Can you work these out from the model? Positions are in its coordinate system, mm. Coordinates: 2 decimals unless noted, no trailing zeros. Write each loop counter-clockwise with the first axis right and the second up, starting at its lowest first coordinate (ties: lowest second). Pieces come first, ordered by that corner, then holes. Notation, with made-up numbers: (37.25, 38) - (57.25, 38) arc R15 cw to (57.25, 47) - close; hole circle Ø4 at (42, -7.5). An arc over 180 degrees is marked (long way). Use one line per item in the form item = value. Start each with the question number.
(1) For pin 1 Ø2 at (x, z) = (-302, -1) entering from +Y; pin 2 Ø14 at (y, z) = (840.5, 18) entering from +X; pin 3 Ø12 at (x, y) = (189.5, 486) entering from +Z; pin 4 Ø2 at (y, z) = (-546.5, 37) entering from +X, each with a flat end and sliding along its axis, tell me the tip position at first contact or that it passes through.
(2) If we section it at A-A on y = -338.5: Please give me the cut outline in (x, z).
(3) If we section it at B-B on z = 18: Give the number of separate pieces and of enclosed holes in the cut face, then the cut area to 3 significant figures.
(4) Thinking about a two-plate mould opening in Y: for faces 1 (the face through (-4, 17, 0)), 2 (the face through (-4, 17, -2)), which applies, pulls with the +Y half, pulls with the -Y half, needs draft (parallel to the pull), parting line crosses it, or undercut?
(5) If we section it at C-C on x = 154: Please give me the cut outline in (y, z), then the cut area to 3 significant figures.
(6) If I drill on probe 1 along X at (y, z) = (146, 30); probe 2 along Y at (x, z) = (214.5, 6); probe 3 along X at (y, z) = (1013, 0.5), over which ranges is the centre line in solid material (lowest first)? Write a range as from..to.
```python
from build123d import *

# Parameters (mm, degrees)
SKETCH1_W                      = 608
SKETCH1_H                      = 2432
BASE_FLANGE1_DEPTH             = 2
EDGE_FLANGE5_STRIP_W           = 13
EDGE_FLANGE5_STRIP_H           = 2
EDGE_FLANGE5_STRIP_CUT_DEPTH   = 608
EDGE_FLANGE5_STRIP_2_W         = 13
EDGE_FLANGE5_STRIP_2_H         = 2
EDGE_FLANGE5_STRIP_CUT_2_DEPTH = 608
EDGE_FLANGE5_DEPTH             = 608
EDGE_FLANGE5_BEND_DEPTH        = 608
EDGE_FLANGE1_STRIP_W           = 13
EDGE_FLANGE1_STRIP_H           = 2
EDGE_FLANGE1_STRIP_CUT_DEPTH   = 2423
EDGE_FLANGE1_STRIP_2_W         = 13
EDGE_FLANGE1_STRIP_2_H         = 2
EDGE_FLANGE1_STRIP_CUT_2_DEPTH = 2423
EDGE_FLANGE1_DEPTH             = 2423
EDGE_FLANGE1_BEND_DEPTH        = 2423
EDGE_FLANGE3_STRIP_W           = 9.4732
EDGE_FLANGE3_STRIP_H           = 2
EDGE_FLANGE3_STRIP_CUT_DEPTH   = 2423
EDGE_FLANGE3_STRIP_2_W         = 9.4732
EDGE_FLANGE3_STRIP_2_H         = 2
EDGE_FLANGE3_STRIP_CUT_2_DEPTH = 2423
EDGE_FLANGE3_DEPTH             = 2423
EDGE_FLANGE3_BEND_DEPTH        = 2423
SKETCH35_R                     = 6
CUT_EXTRUDE1_DEPTH             = 1361.060292781
LPATTERN1_COUNT                = 16
LPATTERN1_PITCH                = 152
SKETCH37_R                     = 6
CUT_EXTRUDE3_DEPTH             = 2754.099344375
LPATTERN3_COUNT                = 4
LPATTERN3_PITCH                = 152


# Sheet-metal steps are written as plain solids
with BuildPart() as part:
    # Sketch1 → Base-Flange1 (new body)
    with BuildSketch(Plane.XY):
        Rectangle(SKETCH1_W, SKETCH1_H)
    extrude(amount=-BASE_FLANGE1_DEPTH)

    # Edge-Flange5 strip (across the edge) → Edge-Flange5 strip cut (cut)
    with BuildSketch(Plane(origin=(304, 1216, 0), x_dir=(0, -1, 0), z_dir=(-1, 0, 0))):
        with Locations((-2, -1)):
            Rectangle(EDGE_FLANGE5_STRIP_W, EDGE_FLANGE5_STRIP_H)
    extrude(amount=EDGE_FLANGE5_STRIP_CUT_DEPTH, mode=Mode.SUBTRACT)

    # Edge-Flange5 strip 2 (across the edge) → Edge-Flange5 strip cut 2 (cut)
    with BuildSketch(Plane(origin=(-304, -1216, 0), x_dir=(0, 1, 0), z_dir=(1, 0, 0))):
        with Locations((-2, -1)):
            Rectangle(EDGE_FLANGE5_STRIP_2_W, EDGE_FLANGE5_STRIP_2_H)
    extrude(amount=EDGE_FLANGE5_STRIP_CUT_2_DEPTH, mode=Mode.SUBTRACT)

    # Edge-Flange5 section (across the edge) → Edge-Flange5 (add)
    with BuildSketch(Plane(origin=(304, 1216, 0), x_dir=(0, -1, 0), z_dir=(-1, 0, 0))):
        with BuildLine():
            Line((0, 2.5), (0, 38))
            Line((0, 38), (2, 38))
            Line((2, 38), (2, 2.5))
            ThreePointArc((2, 2.5), (2.732233047, 0.732233047), (4.5, 0))
            Line((4.5, 0), (4.5, -2))
            ThreePointArc((4.5, -2), (1.318019485, -0.681980515), (0, 2.5))
        make_face()
    extrude(amount=EDGE_FLANGE5_DEPTH)

    # Edge-Flange5 section 2 (across the edge) → Edge-Flange5 bend (add)
    with BuildSketch(Plane(origin=(-304, -1216, 0), x_dir=(0, 1, 0), z_dir=(1, 0, 0))):
        with BuildLine():
            Line((0, 2.5), (0, 38))
            Line((0, 38), (2, 38))
            Line((2, 38), (2, 2.5))
            ThreePointArc((2, 2.5), (2.732233047, 0.732233047), (4.5, 0))
            Line((4.5, 0), (4.5, -2))
            ThreePointArc((4.5, -2), (1.318019485, -0.681980515), (0, 2.5))
        make_face()
    extrude(amount=EDGE_FLANGE5_BEND_DEPTH)

    # Edge-Flange1 strip (across the edge) → Edge-Flange1 strip cut (cut)
    with BuildSketch(Plane(origin=(304, -1211.5, 0), x_dir=(-1, 0, 0), z_dir=(0, 1, 0))):
        with Locations((-2, -1)):
            Rectangle(EDGE_FLANGE1_STRIP_W, EDGE_FLANGE1_STRIP_H)
    extrude(amount=EDGE_FLANGE1_STRIP_CUT_DEPTH, mode=Mode.SUBTRACT)

    # Edge-Flange1 strip 2 (across the edge) → Edge-Flange1 strip cut 2 (cut)
    with BuildSketch(Plane(origin=(-304, 1211.5, 0), x_dir=(1, 0, 0), z_dir=(0, -1, 0))):
        with Locations((-2, -1)):
            Rectangle(EDGE_FLANGE1_STRIP_2_W, EDGE_FLANGE1_STRIP_2_H)
    extrude(amount=EDGE_FLANGE1_STRIP_CUT_2_DEPTH, mode=Mode.SUBTRACT)

    # Edge-Flange1 section (across the edge) → Edge-Flange1 (add)
    with BuildSketch(Plane(origin=(304, -1211.5, 0), x_dir=(-1, 0, 0), z_dir=(0, 1, 0))):
        with BuildLine():
            Line((0, 2.5), (0, 38))
            Line((0, 38), (2, 38))
            Line((2, 38), (2, 2.5))
            ThreePointArc((2, 2.5), (2.732233047, 0.732233047), (4.5, 0))
            Line((4.5, 0), (4.5, -2))
            ThreePointArc((4.5, -2), (1.318019485, -0.681980515), (0, 2.5))
        make_face()
    extrude(amount=EDGE_FLANGE1_DEPTH)

    # Edge-Flange1 section 2 (across the edge) → Edge-Flange1 bend (add)
    with BuildSketch(Plane(origin=(-304, 1211.5, 0), x_dir=(1, 0, 0), z_dir=(0, -1, 0))):
        with BuildLine():
            Line((0, 2.5), (0, 38))
            Line((0, 38), (2, 38))
            Line((2, 38), (2, 2.5))
            ThreePointArc((2, 2.5), (2.732233047, 0.732233047), (4.5, 0))
            Line((4.5, 0), (4.5, -2))
            ThreePointArc((4.5, -2), (1.318019485, -0.681980515), (0, 2.5))
        make_face()
    extrude(amount=EDGE_FLANGE1_BEND_DEPTH)

    # Edge-Flange3 strip (across the edge) → Edge-Flange3 strip cut (cut)
    with BuildSketch(Plane(origin=(302, -1211.5, 38), x_dir=(0, 0, -1), z_dir=(0, 1, 0))):
        with Locations((-2, -1)):
            Rectangle(EDGE_FLANGE3_STRIP_W, EDGE_FLANGE3_STRIP_H)
    extrude(amount=EDGE_FLANGE3_STRIP_CUT_DEPTH, mode=Mode.SUBTRACT)

    # Edge-Flange3 strip 2 (across the edge) → Edge-Flange3 strip cut 2 (cut)
    with BuildSketch(Plane(origin=(-302, 1211.5, 38), x_dir=(0, 0, -1), z_dir=(0, -1, 0))):
        with Locations((-2, -1)):
            Rectangle(EDGE_FLANGE3_STRIP_2_W, EDGE_FLANGE3_STRIP_2_H)
    extrude(amount=EDGE_FLANGE3_STRIP_CUT_2_DEPTH, mode=Mode.SUBTRACT)

    # Edge-Flange3 section (across the edge) → Edge-Flange3 (add)
    with BuildSketch(Plane(origin=(302, -1211.5, 38), x_dir=(0, 0, -1), z_dir=(0, 1, 0))):
        with BuildLine():
            Line((0, 0.7366), (0, 13))
            Line((0, 13), (2, 13))
            Line((2, 13), (2, 0.7366))
            ThreePointArc((2, 0.7366), (2.215745145, 0.215745145), (2.7366, 0))
            Line((2.7366, 0), (2.7366, -2))
            ThreePointArc((2.7366, -2), (0.801531583, -1.198468417), (0, 0.7366))
        make_face()
    extrude(amount=EDGE_FLANGE3_DEPTH)

    # Edge-Flange3 section 2 (across the edge) → Edge-Flange3 bend (add)
    with BuildSketch(Plane(origin=(-302, 1211.5, 38), x_dir=(0, 0, -1), z_dir=(0, -1, 0))):
        with BuildLine():
            Line((0, 0.7366), (0, 13))
            Line((0, 13), (2, 13))
            Line((2, 13), (2, 0.7366))
            ThreePointArc((2, 0.7366), (2.215745145, 0.215745145), (2.7366, 0))
            Line((2.7366, 0), (2.7366, -2))
            ThreePointArc((2.7366, -2), (0.801531583, -1.198468417), (0, 0.7366))
        make_face()
    extrude(amount=EDGE_FLANGE3_BEND_DEPTH)

    # Sketch35 → Cut-Extrude1 (cut, through all)
    with BuildSketch(Plane(origin=(304, 0, 0), x_dir=(0, 0, -1), z_dir=(1, 0, 0))):
        with Locations((-18, -1135.5)):
            Circle(SKETCH35_R)
    cut_extrude1 = extrude(amount=-CUT_EXTRUDE1_DEPTH, mode=Mode.SUBTRACT)

    # LPattern1: Cut-Extrude1 ×16
    with Locations(*[(0, i * LPATTERN1_PITCH, 0) for i in range(1, LPATTERN1_COUNT)]):
        add(cut_extrude1, mode=Mode.SUBTRACT)

    # Sketch37 → Cut-Extrude3 (cut, through all)
    with BuildSketch(Plane(origin=(0, 1216, -1216), x_dir=(1, 0, 0), z_dir=(0, -1, 0))):
        with Locations(Location((228, 1234, 0), (0, 0, 90))):
            Circle(SKETCH37_R)
    cut_extrude3 = extrude(amount=CUT_EXTRUDE3_DEPTH, mode=Mode.SUBTRACT)

    # LPattern3: Cut-Extrude3 ×4
    with Locations(*[(-i * LPATTERN3_PITCH, 0, 0) for i in range(1, LPATTERN3_COUNT)]):
        add(cut_extrude3, mode=Mode.SUBTRACT)


solid = part.part
```
Reported:
q1.pin_1 = 1215.24
q1.pin_2 = 304
q1.pin_3 = 0
q1.pin_4 = 303.9
q2.outline = (-304, 2.5) arc R4.5 ccw to (-299.5, -2) - (299.5, -2) arc R4.5 ccw to (304, 2.5) - (304, 35.26) arc R2.74 ccw to (301.26, 38) - (289, 38) - (289, 36) - (301.26, 36) arc R0.74 cw to (302, 35.26) - (302, 2.5) arc R2.5 cw to (299.5, 0) - (-299.5, 0) arc R2.5 cw to (-302, 2.5) - (-302, 35.26) arc R0.74 cw to (-301.26, 36) - (-289, 36) - (-289, 38) - (-301.26, 38) arc R2.74 ccw to (-304, 35.26) - close
q3.separate_pieces = 44
q3.enclosed_holes = 0
q3.area = 11,200 mm2
q4.face_1 = undercut
q4.face_2 = needs draft
q5.outline = (-1216, 2.5) arc R4.5 ccw to (-1211.5, -2) - (1211.5, -2) arc R4.5 ccw to (1216, 2.5) - (1216, 38) - (1214, 38) - (1214, 2.5) arc R2.5 cw to (1211.5, 0) - (-1211.5, 0) arc R2.5 cw to (-1214, 2.5) - (-1214, 38) - (-1216, 38) - close
q5.area = 5,010 mm2
q6.probe_1 = -304..-302, 302..304
q6.probe_2 = -1216..-1214, 1214..1216
q6.probe_3 = -303.53..-301, 301..303.53
